Autodesk Inventor part; units mm, degrees
ref_plane "YZ Plane" through (0, 0, 0) normal (1, 0, 0) x (0, 1, 0)
ref_plane "XZ Plane" through (0, 0, 0) normal (0, 1, 0) x (-1, 0, 0)
ref_plane "XY Plane" through (0, 0, 0) normal (0, 0, 1) x (1, 0, 0)
sketch "Sketch1" plane through (0, 0, 0) normal (0, 1, 0) x (-1, 0, 0)
  circle A0 centre (0, 0) radius 12.5
  circle A1 centre (0, 0) radius 16.75
  dimension "d0" = 25
  dimension "d1" = 33.5
extrude "Extrusion1" add sketch "Sketch1" along normal blind 3
sketch "Sketch2" plane through (0, 0, 0) normal (0, -1, 0) x (1, 0, 0)
  circle A0 centre (0, 0) radius 12.5
  circle A1 centre (0, 0) radius 12.5
  dimension "d6" = 25
extrude "Extrusion2" add sketch "Sketch2" against normal blind 6.5
fillet "Fillet1" radius 1.5 1 edges at (-12.5, 6.5, 0)
fillet "Fillet2" radius 2.95 1 edges at (16.75, 3, 0)
sketch "Sketch5" plane through (0, 0, 0) normal (0, -1, 0) x (1, 0, 0)
  circle A0 centre (0, 0) radius 16.75
  circle A1 centre (0, 0) radius 14.75
  dimension "d23" = 29.5
extrude "Extrusion5" add sketch "Sketch5" along normal blind 15 contours A1
sketch "Sketch7" plane through (0, -15, 0) normal (0, -1, 0) x (1, 0, 0)
  line L0 (4.9559, 9.4025) -> (-5.0441, 9.4025)
  line L1 (-5.0441, 9.4025) -> (-5.0441, -10.5975)
  line L2 (-5.0441, -10.5975) -> (4.9559, -10.5975)
  line L3 (4.9559, -10.5975) -> (4.9559, 9.4025)
  point P0 (0, 0)
  dimension "d30" = 10
  dimension "d32" = 20
extrude "Extrusion7" add sketch "Sketch7" along normal blind 8
sketch "Sketch8" plane through (0, -23, 0) normal (0, -1, 0) x (1, 0, 0)
  line L0 (-1.0467, 9.4141) -> (2.9533, 9.4141)
  line L1 (2.9533, 9.4141) -> (2.9533, -10.5859)
  line L2 (2.9533, -10.5859) -> (-1.0467, -10.5859)
  line L3 (-1.0467, -10.5859) -> (-1.0467, 9.4141)
  point P0 (0, 0)
  dimension "d35" = 4
  dimension "d37" = 20
extrude "Extrusion8" add sketch "Sketch8" along normal blind 3
sketch "Sketch10" plane through (0, -26, 0) normal (0, -1, 0) x (1, 0, 0)
  line L0 (0.0695, 9.4148) -> (2.0695, 9.4148)
  line L1 (2.0695, 9.4148) -> (2.0695, -10.5852)
  line L2 (2.0695, -10.5852) -> (0.0695, -10.5852)
  line L3 (0.0695, -10.5852) -> (0.0695, 9.4148)
  point P0 (0, 0)
  dimension "d46" = 20
  dimension "d48" = 2
extrude "Extrusion10" add sketch "Sketch10" along normal blind 6
fillet "Fillet3" radius 1 1 edges at (-14.75, -15, 0)
properties part number "OBSF-30-B_button" material "Nylon 6"
Can you work these out from the model? Positions are in its coordinate system, mm. A direction names the side the tool comes from. Give positions to 0.01 mm unless a question says otherwise; leave off trailing zeros. Order: outer loops, then holes, each group sorted by start corner. A loop starts at its lowest first (then second) coordinate and runs counter-clockwise, first axis right, second up. Notation, with made-up numbers: M 79.5,1 L 100.5,1 A13 ccw 100.5,8 Z; hole C -7.5,80 d4. An arc over 180 degrees is marked long. Use one line per item in the form item = value. Start each with the question number.
Item 1: If we section it at C-C (y = -27.5): Write out the boundary of the cut face in (x, z), then the cut area to 3 significant figures.
Item 2: For faces 1 (the flat face through (3.1, 3, 12.3)), 2 (the flat face through (-0.4, -26, -0.4)), 3 (the flat face through (0.07, -29, -1)), 4 (the flat face through (0, -19, -10.598)), which set-ups out of +Z, -Z, +X, -X, +Y, -Y let a thin tool reach every point of the face, with its end or its side?
Item 3: If I drill on line 1 along Y through (x, z) = (-1.5, 5); line 2 along Y through (x, z) = (-7, -7); line 3 along X through (y, z) = (-16, -10.5), over which ranges is the centre line in solid material (lowest first)?
Item 4: If we section it at B-B (y = -18): Write out the boundary of the cut face in (x, z), then the cut area to 3 significant figures.
Item 5: Will these pins go through, and if not, where does the flat tip stop? pin 1 Ø3 at (x, z) = (13, 2.5) entering from +Y; pin 2 Ø10 at (x, y) = (-9.5, -17.5) entering from +Z; pin 3 Ø1.5 at (x, y) = (2, -24) entering from +Z; pin 4 Ø1 at (y, z) = (-17, 12) entering from +X.
Outcome:
q1.outline = M 0.07,-10.59 L 2.07,-10.59 L 2.07,9.41 L 0.07,9.41 Z
q1.area = 40.0 mm2
q2.face_1 = +Y
q2.face_2 = +Z, -Z, -Y
q2.face_3 = +Z, -Z, -X, -Y
q2.face_4 = -Z, +X, -X, -Y
q3.line_1 = -23 to 6.5
q3.line_2 = -15 to 6.5
q3.line_3 = -5.04 to 4.96
q4.outline = M -5.04,-10.6 L 4.96,-10.6 L 4.96,9.4 L -5.04,9.4 Z
q4.area = 200 mm2
q5.pin_1 = 6.31
q5.pin_2 = 13.57
q5.pin_3 = 9.41
q5.pin_4 = through
